Input: part model. Units: mm. Frame: model coordinates. Face numbers are marked on the shaded views. A direction names the side the tool comes from. Give positions to 0.01 mm unless a question says otherwise; leave off trailing zeros. Loops run counter-clockwise (first coordinate to the right, second up) from the corner with the lowest first, then second, coordinate; pieces in that order, holes last. Notation, with made-up numbers: M 51.5,74.5 L 85.5,74.5 A15 ccw 85.5,97.5 Z; hole C -20,-1 d9. An arc over 180 degrees is marked long. Use CSV: the item, a comma, the result in double quotes. Start each with the question number.
from build123d import *

# Parameters (mm, degrees)
SKETCH_1_R             = 5.5
EXTRUDE_1_DEPTH        = 68
CHAMFER_1_SIZE         = 0.5
SKETCH_2_R             = 3.3
EXTRUDE_2_DEPTH        = 8
CHAMFER_2_SIZE         = 0.5
HOLE_WIZARD_M5_1_D     = 4.2
HOLE_WIZARD_M5_1_DEPTH = 12.4
HOLE_WIZARD_M5_1_TIP   = 1.2618073
CHAMFER_3_SIZE         = 0.5
SKETCH_6_W             = 10
SKETCH_6_H             = 3
CUT_EXTRUDE_1_DEPTH    = 13


with BuildPart() as part:
    # 草图1 → 拉伸1 (new body)
    with BuildSketch(Plane.XY):
        Circle(SKETCH_1_R)
    extrude(amount=EXTRUDE_1_DEPTH)

    # 倒角1
    chamfer_1_edges = [part.edges().sort_by_distance(p)[0] for p in [
        (-5.5, 0, 0),
        (-5.5, 0, 68),
    ]]
    chamfer(chamfer_1_edges, length=CHAMFER_1_SIZE)

    # 草图2 → 拉伸2 (add)
    with BuildSketch(Plane.XY.offset(68)):
        Circle(SKETCH_2_R)
    extrude(amount=EXTRUDE_2_DEPTH)

    # 倒角2
    chamfer_2_edges = [part.edges().sort_by_distance(p)[0] for p in [
        (-3.3, 0, 76),
    ]]
    chamfer(chamfer_2_edges, length=CHAMFER_2_SIZE)

    # M5 螺纹孔1
    with Locations(Plane(origin=(0, 0, 0), x_dir=(-1, 0, 0), z_dir=(0, 0, -1))):
        with Locations((0, 0)):
            Hole(HOLE_WIZARD_M5_1_D / 2, depth=HOLE_WIZARD_M5_1_DEPTH)
            with Locations((0, 0, -(HOLE_WIZARD_M5_1_DEPTH + HOLE_WIZARD_M5_1_TIP / 2))):  # 118° drill point
                Cone(0, HOLE_WIZARD_M5_1_D / 2, HOLE_WIZARD_M5_1_TIP, mode=Mode.SUBTRACT)

    # 倒角3
    chamfer_3_edges = [part.edges().sort_by_distance(p)[0] for p in [
        (-2.1, 0, 0),
    ]]
    chamfer(chamfer_3_edges, length=CHAMFER_3_SIZE)

    # 草图6 → 切除-拉伸1 (cut)
    with BuildSketch(Plane(origin=(0, 0, 0), x_dir=(-1, 0, 0), z_dir=(0, 0, -1))):
        with Locations((0, 6.5)):
            Rectangle(SKETCH_6_W, SKETCH_6_H)
        with Locations((0, -6.5)):
            Rectangle(SKETCH_6_W, SKETCH_6_H)
    extrude(amount=-CUT_EXTRUDE_1_DEPTH, mode=Mode.SUBTRACT)


solid = part.part
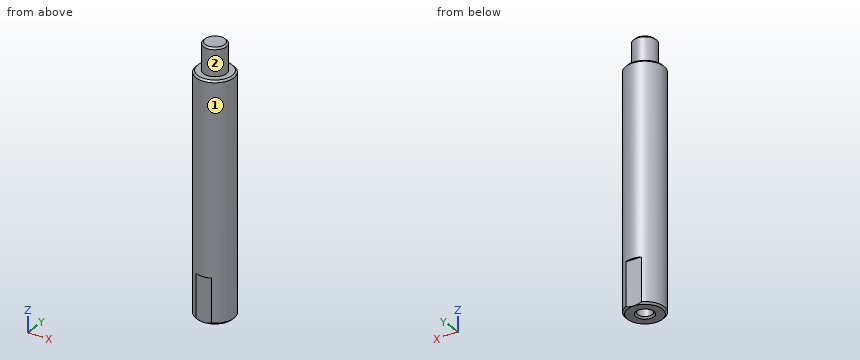
Item 1: Section A-A (z = 6). Output: boundary loops of the cut face in (x, y).
Item 2: Set-up query: the marked faces 1 and 2. Return all of +Z, -Z, +X, -X, +Y, -Y with unobstructed straight access to the full face (end or side cutting, diameter ignored); none if empty.
Item 3: Material intervals for line 1 (X direction, y = 0, z = 9.5); line 2 (Y direction, x = 0, z = 5); line 3 (Z direction, x = -3.75, y = -3), sorted ascending.
Item 4: First-contact query: pin 1 Ø4 at (x, y) = (0, 0) entering from -Z; pin 2 Ø5 at (y, z) = (1.5, 47) entering from -X; pin 3 Ø6 at (x, y) = (-4, 4.5) entering from +Z; pin 4 Ø2 at (x, z) = (4, 39.5) entering from +Y. Flat tips, straight axial feed; report the tip coordinate or a pass-through.
Item 5: Section B-B (z = 55). Output: boundary loops of the cut face in (x, y).
Recorded:
1,outline,"M -2.29,-5 L 2.29,-5 A5.5 ccw 2.29,5 L -2.29,5 A5.5 ccw Z; hole C 0,0 d4.2"
2,face 1,"+Z, -Z"
2,face 2,"+Z"
3,line 1,"-5.5 to -2.1, 2.1 to 5.5"
3,line 2,"-5 to -2.1, 2.1 to 5"
3,line 3,"0 to 68"
4,pin 1,"z = 12.46"
4,pin 2,"x = -5.5"
4,pin 3,"z = 75.78"
4,pin 4,"y = 4.61"
5,outline,"C 0,0 d11"
